Check sheet for the modelled part. Datum: model origin and axes. Units: mm. Round coordinates to 2 decimals unless told otherwise and drop trailing zeros. Loops run counter-clockwise (first coordinate to the right, second up) from the corner with the lowest first, then second, coordinate; pieces in that order, holes last. Notation, with made-up numbers: (20, 27.25) -> (61, 27.25) arc R10 ccw to (61, 44.25) -> close; hole circle Ø6 at (53, 63.25). An arc over 180 degrees is marked (long way). Use one line per item in the form item = value. Start each with the question number.
(1) Sectioned sample at D-D (x = -49). Record the cut outline in (y, z).
(2) Material ranges on probe 1 along X at (y, z) = (6, 0.65); probe 2 along X at (y, z) = (99, 0.9); probe 3 along X at (y, z) = (19.05, 2.1), recorded low to high. Write a range as [from, to].
(3) Go/stop test with flat-tipped pins: pin 1 (3 mm diameter, centred on x = 91.09, y = -44.13, fed in from -Z); pin 2 (5.5 mm diameter, centred on x = 95.62, y = -33.21, fed in from +Z); pin 3 (3 mm diameter, centred on x = -10.5, z = 3, fed in from -Y). Record where each tip stops, or that it passes through.
(4) Sectioned sample at C-C (z = 3.55). State how many separate pieces and enclosed holes the cut face has, and give its area (3 significant figures).
(5) Sectioned sample at A-A (y = 0). Record the cut outline in (x, z), and give its area (3 significant figures).
from build123d import *

# Parameters (mm, degrees)
F0_R            = 114.6499739
F0_R_2          = 1.7272
F0_R_3          = 12.7
F1_DEPTH        = 5.08
F2_R            = 1.7272
F3_DEPTH        = 5.08
F3_COPIES_COUNT = 24


# Not quite as in the source:
# - a pattern or mirror of a feature is missing from the dataset's text; its kind, count and spacing are read off the source's solid


with BuildPart() as f1:
    # F0 (on Top) → F1 (new body)
    with BuildSketch(Plane.XY):
        Circle(F0_R)
        with Locations((-12.909118174, -12.909118174)):
            Circle(F0_R_2, mode=Mode.SUBTRACT)
        with Locations((12.909118174, -12.909118174)):
            Circle(F0_R_2, mode=Mode.SUBTRACT)
        with Locations((-12.909118174, 12.909118174)):
            Circle(F0_R_2, mode=Mode.SUBTRACT)
        Circle(F0_R_3, mode=Mode.SUBTRACT)
        with Locations((12.909118174, 12.909118174)):
            Circle(F0_R_2, mode=Mode.SUBTRACT)
    extrude(amount=F1_DEPTH)

    # F2 (on face) → F3 (cut, through all)
    with BuildSketch(Plane.XY.offset(5.08)):
        with Locations((19.05, -99.4099739)):
            Circle(F2_R)
        with Locations((-19.05, -99.4099739)):
            Circle(F2_R)
    f3 = extrude(amount=-F3_DEPTH, mode=Mode.SUBTRACT)

    # F3_copies: F3 ×24 about axis
    f3_copies_axis = Axis((0, 0, 0), (0, 0, 1))
    for i in range(1, F3_COPIES_COUNT):
        add(f3.rotate(f3_copies_axis, i * 360 / F3_COPIES_COUNT), mode=Mode.SUBTRACT)


solid = f1.part
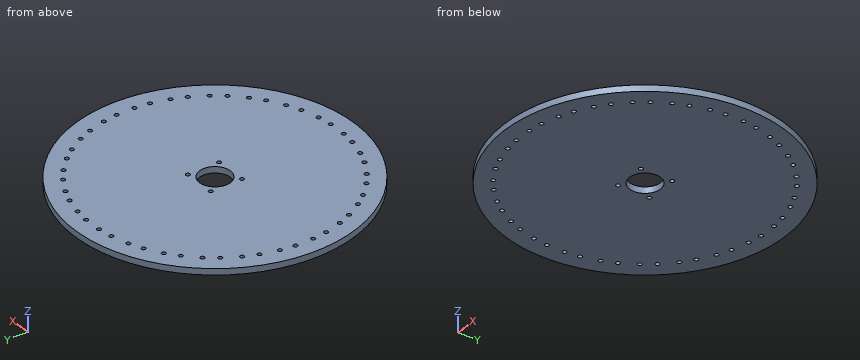
Checks:
q1.outline = (-103.65, 0) -> (103.65, 0) -> (103.65, 5.08) -> (-103.65, 5.08) -> close
q2.probe_1 = [-114.49, -102.06], [-99.85, -11.19], [11.19, 99.85], [102.06, 114.49]
q2.probe_2 = [-57.82, -20.73], [-17.37, 17.37], [20.73, 57.82]
q2.probe_3 = [-113.06, -101.14], [-97.68, 97.68], [101.14, 113.06]
q3.pin_1 = through
q3.pin_2 = 5.08
q3.pin_3 = -114.3
q4.separate_pieces = 1
q4.enclosed_holes = 53
q4.area = 40,300 mm2
q5.outline = (-114.65, 0) -> (-12.7, 0) -> (-12.7, 5.08) -> (-114.65, 5.08) -> close; (12.7, 0) -> (114.65, 0) -> (114.65, 5.08) -> (12.7, 5.08) -> close
q5.area = 1,040 mm2
